from build123d import *

# Parameters (mm, degrees)
SKETCH1_R           = 32.5
BOSS_EXTRUDE1_DEPTH = 7
SKETCH2_R           = 3.5
SKETCH2_R_2         = 1
CUT_EXTRUDE1_DEPTH  = 10
SKETCH3_R           = 35.5
CUT_EXTRUDE2_DEPTH  = 6
FILLET1_R           = 10
SKETCH4_R           = 1.5
CUT_EXTRUDE3_DEPTH  = 10
SKETCH5_R           = 3.5
SKETCH5_R_2         = 1.5
BOSS_EXTRUDE2_DEPTH = 6
SKETCH6_R           = 3
CUT_EXTRUDE4_DEPTH  = 4
SKETCH8_R           = 3
SKETCH8_R_2         = 1
BOSS_EXTRUDE3_DEPTH = 3
SKETCH9_R           = 35.5
SKETCH9_R_2         = 31.5
BOSS_EXTRUDE4_DEPTH = 1


with BuildPart() as part:
    # Sketch1 → Boss-Extrude1 (new body)
    with BuildSketch(Plane.XZ.offset(-37.073034342)):
        with BuildLine():
            ThreePointArc((38.4, -11.2), (39.923628268, 2.470608411), (36.72611339, 15.849056604))
            Line((36.72611339, 15.849056604), (17.44490386, 60.528301887))
            ThreePointArc((17.44490386, 60.528301887), (0, 72), (-17.44490386, 60.528301887))
            Line((-17.44490386, 60.528301887), (-36.72611339, 15.849056604))
            ThreePointArc((-36.72611339, 15.849056604), (-39.923628268, 2.470608411), (-38.4, -11.2))
            Line((-38.4, -11.2), (-30, -40))
            Line((-30, -40), (30, -40))
            Line((30, -40), (38.4, -11.2))
        make_face()
        Circle(SKETCH1_R, mode=Mode.SUBTRACT)
    extrude(amount=-BOSS_EXTRUDE1_DEPTH)

    # Sketch2 → Cut-Extrude1 (cut)
    with BuildSketch(Plane(origin=(0, 44.073034342, 0), x_dir=(1, 0, 0), z_dir=(0, 1, 0))):
        with Locations((0, -53)):
            Circle(SKETCH2_R)
        with Locations((11, -53)):
            Circle(SKETCH2_R_2)
        with Locations((-11, -53)):
            Circle(SKETCH2_R_2)
    extrude(amount=-CUT_EXTRUDE1_DEPTH, mode=Mode.SUBTRACT)

    # Sketch3 → Cut-Extrude2 (cut)
    with BuildSketch(Plane.XZ.offset(-37.073034342)):
        with BuildLine():
            Line((34.889807721, 15.056603774), (15.608598191, 59.735849057))
            ThreePointArc((15.608598191, 59.735849057), (0, 70), (-15.608598191, 59.735849057))
            Line((-15.608598191, 59.735849057), (-34.889807721, 15.056603774))
            ThreePointArc((-34.889807721, 15.056603774), (-37.927446855, 2.347077991), (-36.48, -10.64))
            Line((-36.48, -10.64), (-28.5, -38))
            Line((-28.5, -38), (28.5, -38))
            Line((28.5, -38), (36.48, -10.64))
            ThreePointArc((36.48, -10.64), (37.927446855, 2.347077991), (34.889807721, 15.056603774))
        make_face()
        Circle(SKETCH3_R, mode=Mode.SUBTRACT)
    extrude(amount=-CUT_EXTRUDE2_DEPTH, mode=Mode.SUBTRACT)

    # Fillet1
    fillet1_edges = [part.edges().sort_by_distance(p)[0] for p in [
        (30, 40.573034342, -40),
        (-30, 40.573034342, -40),
        (28.5, 40.073034342, -38),
        (-28.5, 40.073034342, -38),
    ]]
    fillet(fillet1_edges, radius=FILLET1_R)

    # Sketch4 → Cut-Extrude3 (cut)
    with BuildSketch(Plane(origin=(0, 44.073034342, 0), x_dir=(1, 0, 0), z_dir=(0, 1, 0))):
        with Locations((-20, 36)):
            Circle(SKETCH4_R)
        with Locations((20, 36)):
            Circle(SKETCH4_R)
        with Locations((23, -38)):
            Circle(SKETCH4_R)
        with Locations((-23, -38)):
            Circle(SKETCH4_R)
    extrude(amount=-CUT_EXTRUDE3_DEPTH, mode=Mode.SUBTRACT)

    # Sketch5 → Boss-Extrude2 (add)
    with BuildSketch(Plane.XZ.offset(-43.073034342)):
        with Locations((-23, 38)):
            Circle(SKETCH5_R)
        with Locations((-23, 38)):
            Circle(SKETCH5_R_2, mode=Mode.SUBTRACT)
        with Locations((23, 38)):
            Circle(SKETCH5_R)
        with Locations((23, 38)):
            Circle(SKETCH5_R_2, mode=Mode.SUBTRACT)
        with Locations((-20, -36)):
            Circle(SKETCH5_R)
        with Locations((-20, -36)):
            Circle(SKETCH5_R_2, mode=Mode.SUBTRACT)
        with Locations((20, -36)):
            Circle(SKETCH5_R)
        with Locations((20, -36)):
            Circle(SKETCH5_R_2, mode=Mode.SUBTRACT)
    extrude(amount=BOSS_EXTRUDE2_DEPTH)

    # Sketch6 → Cut-Extrude4 (cut)
    with BuildSketch(Plane(origin=(0, 44.073034342, 0), x_dir=(1, 0, 0), z_dir=(0, 1, 0))):
        with Locations((-20, 36)):
            Circle(SKETCH6_R)
        with Locations((20, 36)):
            Circle(SKETCH6_R)
        with Locations((-23, -38)):
            Circle(SKETCH6_R)
        with Locations((23, -38)):
            Circle(SKETCH6_R)
    extrude(amount=-CUT_EXTRUDE4_DEPTH, mode=Mode.SUBTRACT)

    # Sketch8 → Boss-Extrude3 (add)
    with BuildSketch(Plane.XZ.offset(-43.073034342)):
        with Locations((11, 53)):
            Circle(SKETCH8_R)
        with Locations((11, 53)):
            Circle(SKETCH8_R_2, mode=Mode.SUBTRACT)
        with Locations((-11, 53)):
            Circle(SKETCH8_R)
        with Locations((-11, 53)):
            Circle(SKETCH8_R_2, mode=Mode.SUBTRACT)
    extrude(amount=BOSS_EXTRUDE3_DEPTH)

    # Sketch9 → Boss-Extrude4 (add)
    with BuildSketch(Plane.XZ.offset(-37.073034342)):
        Circle(SKETCH9_R)
        Circle(SKETCH9_R_2, mode=Mode.SUBTRACT)
    extrude(amount=BOSS_EXTRUDE4_DEPTH)


solid = part.part
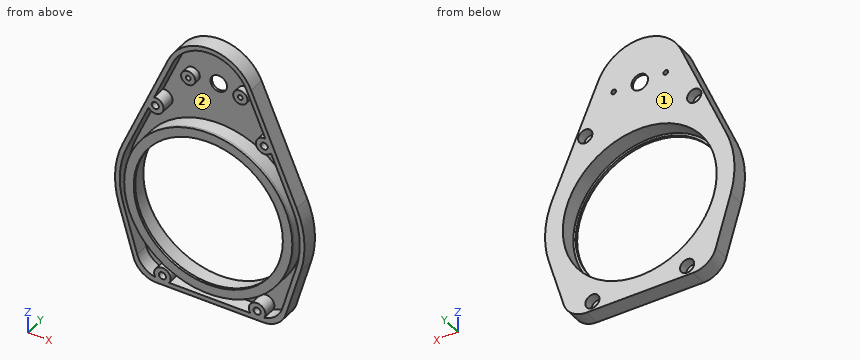
The model under review builds one solid part; all positions refer to its coordinate system, in mm. Face numbers are marked on the shaded views. Round coordinates to 2 decimals unless told otherwise and drop trailing zeros. Loops run counter-clockwise (first coordinate to the right, second up) from the corner with the lowest first, then second, coordinate; pieces in that order, holes last. Notation, with made-up numbers: M 67,79.5 L 113,79.5 A14 cw 113,90.5 Z; hole C -25.5,35 d11. An arc over 180 degrees is marked long. Answer as a JSON object with one key per item and string values.
Item 1: We need section A-A, the plane y = 38.75. State how many separate pieces and enclosed holes the cut face has, and give its area (3 significant figures).
Check sheet entries:
{"separate pieces": "2", "enclosed holes": "6", "area": "1,360 mm2"}
Item 2: We need section C-C, the plane z = 43.5. State the section outline as (x, y) points.
Check sheet entries:
{"outline": "M -24.79,37.07 L -22.62,37.07 L -22.62,43.07 L 22.62,43.07 L 22.62,37.07 L 24.79,37.07 L 24.79,44.07 L -24.79,44.07 Z"}
Item 3: The part is to be moulded in two halves that separate along X. For the marked faces 1 and 2, say which applies: +X half, -X half, draft (parallel to the pull), parting line (faces both ways), or undercut.
Check sheet entries:
{"face 1": "draft", "face 2": "undercut"}
Item 4: We need section D-D, the plane z = -29.5. State the section outline as (x, y) points.
Check sheet entries:
{"outline": "M -33.06,37.07 L -30.98,37.07 L -30.98,43.07 L -19.75,43.07 L -19.75,36.07 L -11.05,36.07 L -11.05,37.07 L -13.64,37.07 L -13.64,44.07 L -33.06,44.07 Z; M 11.05,36.07 L 19.75,36.07 L 19.75,43.07 L 30.98,43.07 L 30.98,37.07 L 33.06,37.07 L 33.06,44.07 L 13.64,44.07 L 13.64,37.07 L 11.05,37.07 Z"}
Item 5: We need section B-B, the plane z = -2.5. State the section outline as (x, y) points.
Check sheet entries:
{"outline": "M -39.92,37.07 L -37.92,37.07 L -37.92,43.07 L -35.41,43.07 L -35.41,36.07 L -31.4,36.07 L -31.4,37.07 L -32.4,37.07 L -32.4,44.07 L -39.92,44.07 Z; M 31.4,36.07 L 35.41,36.07 L 35.41,43.07 L 37.92,43.07 L 37.92,37.07 L 39.92,37.07 L 39.92,44.07 L 32.4,44.07 L 32.4,37.07 L 31.4,37.07 Z"}
Item 6: Clearance check with flat-ended pins moving along their axes: P1, Ø1.8, axis at x = -23, z = 38, coming from the -Y side; P2, Ø4, axis at y = 42, z = 36.5, coming from the -X side; P3, Ø3, axis at x = -11, z = 53, coming from the -Y side; P4, Ø9.5, axis at x = -20, z = -36, coming from the -Y side. State where each tip first meets the part, or that it passes through.
Check sheet entries:
{"P1": "through", "P2": "x = -28.68", "P3": "y = 40.07", "P4": "y = 37.07"}
Item 7: For line 1 along X through (y, z) = (37.5, -0.5); line 2 along Z through (x, y) = (20, 39.3); line 3 along X through (y, z) = (43, 2), list the stretches that pass through material, from the lowest coordinate up.
Check sheet entries:
{"line 1": "-40 to -38, -35.5 to -32.5, 32.5 to 35.5, 38 to 40", "line 2": "-40 to -37.5, -34.5 to -32.5, -29.33 to -25.62, 25.62 to 29.33, 36.2 to 39.8, 49.56 to 54.61", "line 3": "-39.95 to -37.95, -35.44 to -32.44, 32.44 to 35.44, 37.95 to 39.95"}
